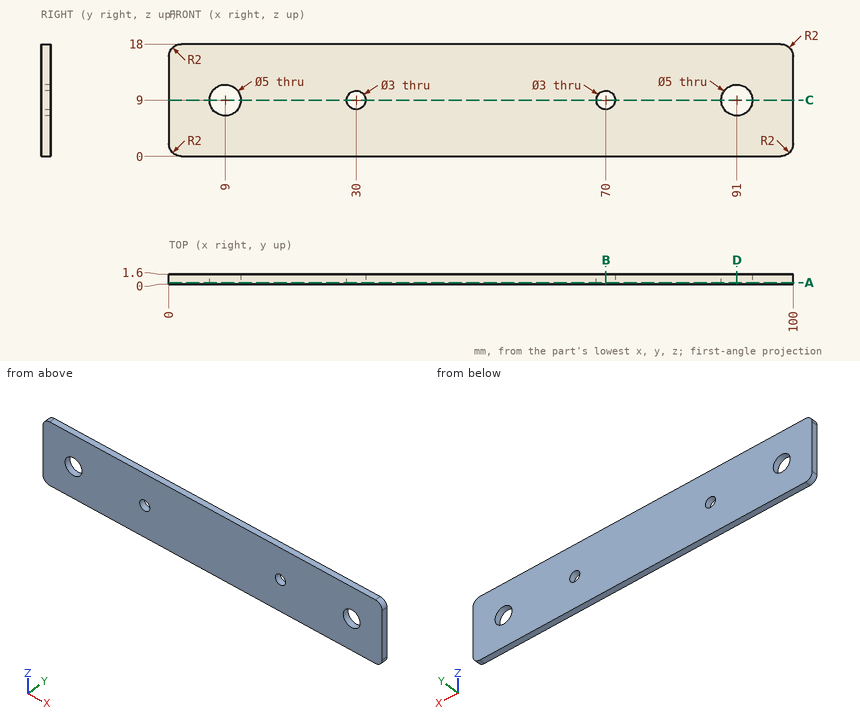
Source: three-view drawing plus pictorial views. Frame: mm from the lowest corner of the part. Coordinates: 2 decimals unless noted, no trailing zeros. Order: outer loops, then holes, each group sorted by start corner. A loop starts at its lowest first (then second) coordinate and runs counter-clockwise, first axis right, second up. Notation, with made-up numbers: M 49,-34 L 59,-34 A20 cw 59,-19 Z; hole C 51.25,42 d2. An arc over 180 degrees is marked long. One line per question, with ' | ' between items. Start each with the question number.
Item 1: Cut plane D-D, the plane x = 91. Return the cut outline in (y, z).
Item 2: Cut plane C-C, the plane z = 9. Return the cut outline in (x, y).
Item 3: Ray query, probe 1 along Z at (x, y) = (70, 0.3); probe 2 along X at (y, z) = (1.2, 11); probe 3 along Z at (x, y) = (9, 0.5). Return the intervals inside material, ascending. Write a range as [from, to].
Item 4: Cut plane A-A, the plane y = 0.25. Return the cut outline in (x, z).
Item 5: Cut plane B-B, the plane x = 70. Return the cut outline in (y, z), then the cut area to 3 significant figures.
A:
1) outline: M 0,0 L 1.6,0 L 1.6,6.5 L 0,6.5 Z; M 0,11.5 L 1.6,11.5 L 1.6,18 L 0,18 Z
2) outline: M 0,0 L 6.5,0 L 6.5,1.6 L 0,1.6 Z; M 11.5,0 L 28.5,0 L 28.5,1.6 L 11.5,1.6 Z; M 31.5,0 L 68.5,0 L 68.5,1.6 L 31.5,1.6 Z; M 71.5,0 L 88.5,0 L 88.5,1.6 L 71.5,1.6 Z; M 93.5,0 L 100,0 L 100,1.6 L 93.5,1.6 Z
3) probe 1: z = [0, 7.5], [10.5, 18] | probe 2: x = [0, 7.5], [10.5, 89.5], [92.5, 100] | probe 3: z = [0, 6.5], [11.5, 18]
4) outline: M 0,2 A2 ccw 2,0 L 98,0 A2 ccw 100,2 L 100,16 A2 ccw 98,18 L 2,18 A2 ccw 0,16 Z; hole C 9,9 d5; hole C 30,9 d3; hole C 70,9 d3; hole C 91,9 d5
5) outline: M 0,0 L 1.6,0 L 1.6,7.5 L 0,7.5 Z; M 0,10.5 L 1.6,10.5 L 1.6,18 L 0,18 Z | area: 24.0 mm2
